The model under review builds one solid part; all positions refer to its coordinate system, in mm. A direction names the side the tool comes from. Coordinates: 2 decimals unless noted, no trailing zeros. Write each loop counter-clockwise with the first axis right and the second up, starting at its lowest first coordinate (ties: lowest second). Pieces come first, ordered by that corner, then holes. Notation, with made-up numbers: (17, 71) -> (21, 71) arc R15 cw to (21, 87) -> close; hole circle Ø3 at (-15.75, -36). An arc over 180 degrees is marked (long way). Put each result on its own line as item: value. Start each with the question number.
from build123d import *

# Parameters (mm, degrees)
F0_W     = 72.716318
F0_H     = 84.215194
F1_DEPTH = 25.4
F2_R     = 23.274409
F3_DEPTH = 50.8
F4_R     = 16.862777
F5_DEPTH = 50.801


with BuildPart() as f1:
    # F0 (on Front) → F1 (new body)
    with BuildSketch(Plane.XZ):
        with Locations((2.836455, -0.9862)):
            Rectangle(F0_W, F0_H)
    extrude(amount=F1_DEPTH)

    # F2 (on Front) → F3 (join)
    with BuildSketch(Plane.XZ):
        Circle(F2_R)
    extrude(amount=F3_DEPTH)

    # F4 (on face) → F5 (cut, through all)
    with BuildSketch(Plane.XZ.offset(50.8)):
        Circle(F4_R)
    extrude(amount=-F5_DEPTH, mode=Mode.SUBTRACT)


solid = f1.part
1. The part is to be moulded in two halves that separate along X. For faces 3 (the cylindrical face through (-18.47, -37.92, -14.16)), 4 (the flat face through (2, -13, 41.121)), 5 (the cylindrical face through (9.065, -25.756, 14.219)), say which applies: released by +X, released by -X, zero draft, split by the parting line, or undercut.
2. Consider section D-D on x = 32. State the section outline as (y, z) points, then the cut area to 3 significant figures.
3. Wall thickness on line 1 (Z direction, x = 0, y = -21.5); line 2 (Y direction, x = 3, z = 34); line 3 (Z direction, x = 0, y = -26): over which ranges is each line inside the solid? List them lowest first. Write a range as from..to.
4. Insertion check: P1, Ø1, axis at x = -14, y = -30.5, coming from the -Z side; P2, Ø4, axis at x = -24.5, z = 22, coming from the +Y side; P3, Ø1, axis at x = 25.5, y = -30, coming from the -Z side; P4, Ø6, axis at y = -44, z = -22.5, coming from the +X side. Each pin has a flat end and moves straight along its axis. Give the tip position at first contact, or say it passes through.
5. Tool access review of faces 1 (the flat face through (39.195, -13, -2)), 2 (the flat face through (27, -25.4, 0)): name each direction out of +Z, -Z, +X, -X, +Y, -Y from which nothing blocks a thin tool from reaching the whole face with its end or side.
6. Consider section B-B on y = -8. State the section outline as (x, z) points, then the cut area to 3 significant figures.
7. Consider section A-A on z = 0. State the section outline as (x, y) points.
8. Consider section C-C on x = 0. State the section outline as (y, z) points.
Output values:
1. face 3: split by the parting line
1. face 4: zero draft
1. face 5: undercut
2. outline: (-25.4, -43.09) -> (0, -43.09) -> (0, 41.12) -> (-25.4, 41.12) -> close
2. area: 2,140 mm^2
3. line 1: z = -43.09..-16.86, 16.86..41.12
3. line 2: y = -25.4..0
3. line 3: z = -23.27..-16.86, 16.86..23.27
4. P1: stops at z = -18.96
4. P2: stops at y = 0
4. P3: passes through
4. P4: stops at x = 12.71
5. face 1: +Z, -Z, +X, +Y, -Y
5. face 2: -Y
6. outline: (-33.52, -43.09) -> (39.19, -43.09) -> (39.19, 41.12) -> (-33.52, 41.12) -> close; hole circle Ø33.73 at (0, 0)
6. area: 5,230 mm^2
7. outline: (-33.52, -25.4) -> (-23.27, -25.4) -> (-23.27, -50.8) -> (-16.86, -50.8) -> (-16.86, 0) -> (-33.52, 0) -> close; (16.86, -50.8) -> (23.27, -50.8) -> (23.27, -25.4) -> (39.19, -25.4) -> (39.19, 0) -> (16.86, 0) -> close
8. outline: (-50.8, -23.27) -> (-25.4, -23.27) -> (-25.4, -43.09) -> (0, -43.09) -> (0, -16.86) -> (-50.8, -16.86) -> close; (-50.8, 16.86) -> (0, 16.86) -> (0, 41.12) -> (-25.4, 41.12) -> (-25.4, 23.27) -> (-50.8, 23.27) -> close
